```python
from build123d import *

# Parameters (mm, degrees)
SKETCH_W      = 50
SKETCH_H      = 50
PAD_DEPTH     = 3
SKETCH001_W   = 10
SKETCH001_H   = 10
POCKET_DEPTH  = 5
SKETCH002_W   = 50
SKETCH002_H   = 50
SKETCH002_W_2 = 46
SKETCH002_H_2 = 46
PAD001_DEPTH  = 50
SKETCH003_W   = 34
SKETCH003_H   = 34
SKETCH003_W_2 = 30
SKETCH003_H_2 = 30
PAD002_DEPTH  = 50


with BuildPart() as part:
    # Sketch → Pad (new body)
    with BuildSketch(Plane.XY):
        with Locations((25, 25)):
            Rectangle(SKETCH_W, SKETCH_H)
    extrude(amount=PAD_DEPTH)

    # Sketch001 (on Face6 of Pad) → Pocket (cut)
    with BuildSketch(Plane.XY.offset(3)):
        with Locations((25, 25)):
            Rectangle(SKETCH001_W, SKETCH001_H)
    extrude(amount=-POCKET_DEPTH, mode=Mode.SUBTRACT)

    # Sketch002 (on Face5 of Pocket) → Pad001 (join)
    with BuildSketch(Plane.XY.offset(3)):
        with Locations((25, 25)):
            Rectangle(SKETCH002_W, SKETCH002_H)
        with Locations((25, 25)):
            Rectangle(SKETCH002_W_2, SKETCH002_H_2, mode=Mode.SUBTRACT)
    extrude(amount=PAD001_DEPTH)

    # Sketch003 (on Face15 of Pad001) → Pad002 (join)
    with BuildSketch(Plane.XY.offset(3)):
        with Locations((25, 25)):
            Rectangle(SKETCH003_W, SKETCH003_H)
        with Locations((25, 25)):
            Rectangle(SKETCH003_W_2, SKETCH003_H_2, mode=Mode.SUBTRACT)
    extrude(amount=PAD002_DEPTH)


solid = part.part
```
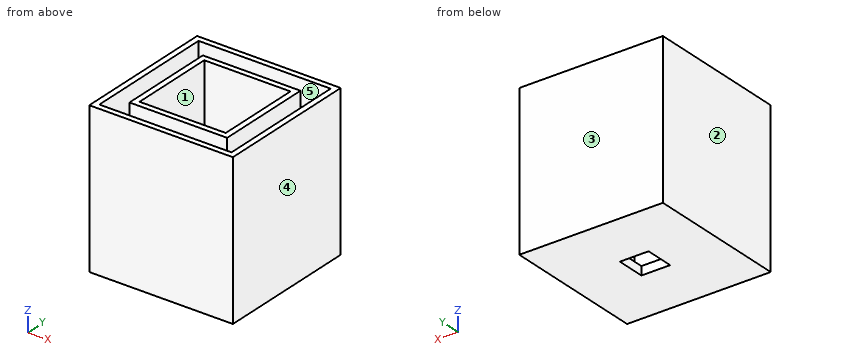
Verification items for the finished model (mm, model axes). Face numbers are marked on the shaded views. A direction names the side the tool comes from. Coordinates: 2 decimals unless noted, no trailing zeros. Loops run counter-clockwise (first coordinate to the right, second up) from the corner with the lowest first, then second, coordinate; pieces in that order, holes last. Notation, with made-up numbers: (56, 23) - (101, 23) arc R25 cw to (101, 38) - close; hole circle Ø10 at (77, 71). An arc over 180 degrees is marked (long way). Answer as a JSON object with one key per item and string values.
(1) Cross-section at A-A, the plane z = 40.5. Record the boundary of the cut face in (x, y).
Response:
{"outline": "(0, 0) - (50, 0) - (50, 50) - (0, 50) - close; (8, 8) - (42, 8) - (42, 42) - (8, 42) - close; hole (2, 2) - (48, 2) - (48, 48) - (2, 48) - close; hole (10, 10) - (40, 10) - (40, 40) - (10, 40) - close"}
(2) Access from +Z, -Z, +X, -X, +Y, -Y to the whole of each face (thin tool, end or side, straight path). Record for the marked faces 1 and 2.
Response:
{"face 1": "+Z", "face 2": "+Z, -Z, -X, +Y, -Y"}
(3) Mould release check, pull along Y, two halves, no side actions. Record for the marked faces 3, 4 and 5: pulls with the +Y half, pulls with the -Y half, needs draft (parallel to the pull), parting line crosses it, or undercut.
Response:
{"face 3": "pulls with the +Y half", "face 4": "needs draft", "face 5": "undercut"}
(4) Cross-section at B-B, the plane x = 25.5. Record the boundary of the cut face in (y, z), then the cut area to 3 significant figures.
Response:
{"outline": "(0, 0) - (20, 0) - (20, 3) - (10, 3) - (10, 53) - (8, 53) - (8, 3) - (2, 3) - (2, 53) - (0, 53) - close; (30, 0) - (50, 0) - (50, 53) - (48, 53) - (48, 3) - (42, 3) - (42, 53) - (40, 53) - (40, 3) - (30, 3) - close", "area": "520 mm²"}
(5) Cross-section at D-D, the plane x = 38. Record the boundary of the cut face in (y, z).
Response:
{"outline": "(0, 0) - (50, 0) - (50, 53) - (48, 53) - (48, 3) - (42, 3) - (42, 53) - (40, 53) - (40, 3) - (10, 3) - (10, 53) - (8, 53) - (8, 3) - (2, 3) - (2, 53) - (0, 53) - close"}
(6) Go/stop test with a flat-tipped pin: pin 1 Ø14 at (x, y) = (29, 19) entering from +Z. Record where the tip stops, or that it passes through.
Response:
{"pin 1": "stops at z = 3"}
(7) Scan lines: line 1 along Y through (x, z) = (13, 9); line 2 along X through (y, z) = (41, 26). Record each from-to range of solid material in increasing order.
Response:
{"line 1": "y = 0 to 2, 8 to 10, 40 to 42, 48 to 50", "line 2": "x = 0 to 2, 8 to 42, 48 to 50"}
